Can you work these out from the drawing? Everything is in mm from the part's minimum corner. A direction names the side the tool comes from. Round coordinates to 2 decimals unless told otherwise and drop trailing zeros. Order: outer loops, then holes, each group sorted by start corner. A loop starts at its lowest first (then second) coordinate and runs counter-clockwise, first axis right, second up. Notation, with made-up numbers: (8.25, 71.5) - (43.25, 71.5) arc R23 ccw to (43.25, 98.5) - close; hole circle Ø8 at (50.5, 21.5). An arc over 180 degrees is marked (long way). Answer as a JSON object with one key per item and string values.
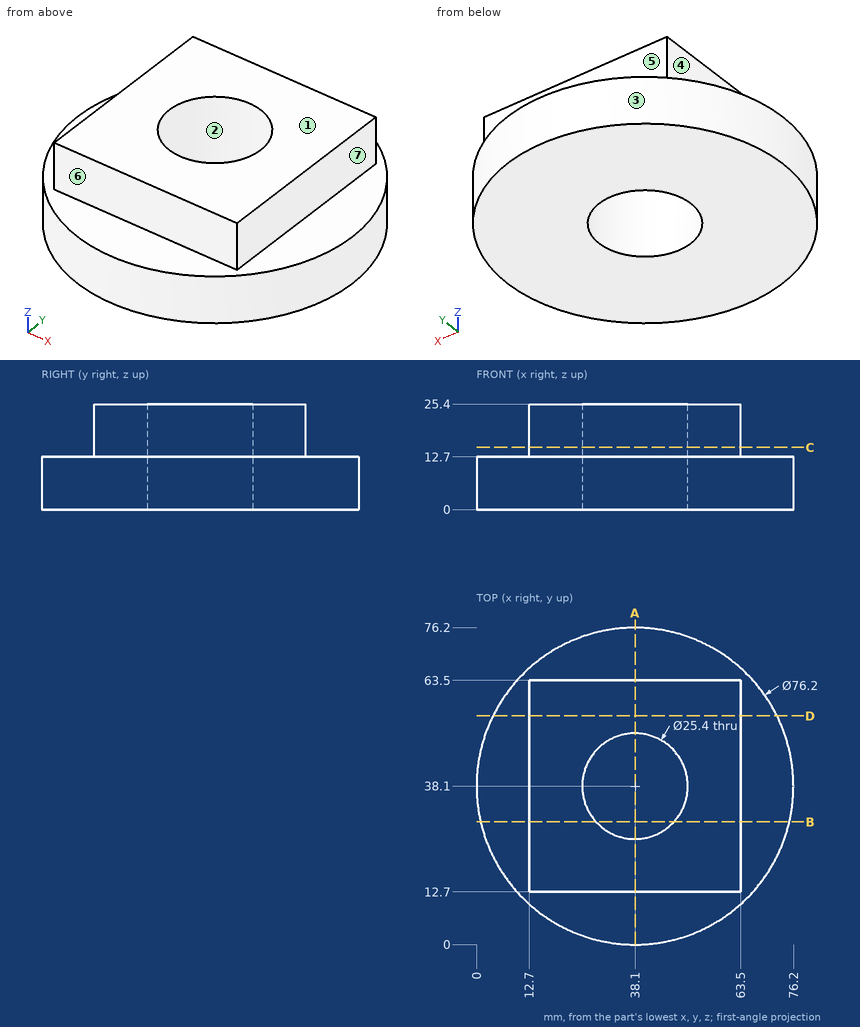
1. Imagine slicing it at A-A (x = 38.1). List the corners of the cut face in (y, z) for me.
Responses:
{"outline": "(0, 0) - (25.4, 0) - (25.4, 25.4) - (12.7, 25.4) - (12.7, 12.7) - (0, 12.7) - close; (50.8, 0) - (76.2, 0) - (76.2, 12.7) - (63.5, 12.7) - (63.5, 25.4) - (50.8, 25.4) - close"}
2. Imagine slicing it at D-D (y = 55). List the corners of the cut face in (x, z) for me.
Responses:
{"outline": "(3.95, 0) - (72.25, 0) - (72.25, 12.7) - (63.5, 12.7) - (63.5, 25.4) - (12.7, 25.4) - (12.7, 12.7) - (3.95, 12.7) - close"}
3. For the marked faces 4, 5, 6 and 7, which set-ups out of +Z, -Z, +X, -X, +Y, -Y let a thin tool reach every point of the face, with its end or its side?
Responses:
{"face 4": "+Z, -X, +Y, -Y", "face 5": "+Z, +X, -X, +Y", "face 6": "+Z, +X, -X, -Y", "face 7": "+Z, +X, +Y, -Y"}
4. Imagine slicing it at C-C (z = 15). List the corners of the cut face in (x, y) for me, plus the area to 3 significant figures.
Responses:
{"outline": "(12.7, 12.7) - (63.5, 12.7) - (63.5, 63.5) - (12.7, 63.5) - close; hole circle Ø25.4 at (38.1, 38.1)", "area": "2,070 mm2"}
5. Imagine slicing it at B-B (y = 29.5). List the corners of the cut face in (x, z) for me.
Responses:
{"outline": "(0.98, 0) - (28.75, 0) - (28.75, 25.4) - (12.7, 25.4) - (12.7, 12.7) - (0.98, 12.7) - close; (47.45, 0) - (75.22, 0) - (75.22, 12.7) - (63.5, 12.7) - (63.5, 25.4) - (47.45, 25.4) - close"}
6. For P1, Ø12, axis at x = 11.5, z = 9.5, coming from the +Y side; P2, Ø1, axis at x = 22, z = 4.5, coming from the +Y side; P3, Ø4, axis at x = 37.5, z = 22, coming from the +Y side; P4, Ø8, axis at x = 9, y = 50.5, coming from the +Z side, each with a flat end and sliding along its axis, tell me the tip position at first contact or that it passes through.
Responses:
{"P1": "y = 70.15", "P2": "y = 72.86", "P3": "y = 63.5", "P4": "z = 25.4"}
7. Thinking about a two-plate mould opening in Y: for the marked faces 1, 2 and 3, which applies, pulls with the +Y half, pulls with the -Y half, needs draft (parallel to the pull), parting line crosses it, or undercut?
Responses:
{"face 1": "needs draft", "face 2": "undercut", "face 3": "parting line crosses it"}
8. If I drill on L1, parallel to X at y = 37.5, z = 19; L2, parallel to Y at x = 38.1, z = 20.25; L3, parallel to Y at x = 47.5, z = 5.5, over which ranges is the centre line in solid material (lowest first)? Write a range as [from, to].
Responses:
{"L1": "[12.7, 25.41], [50.79, 63.5]", "L2": "[12.7, 25.4], [50.8, 63.5]", "L3": "[1.18, 29.56], [46.64, 75.02]"}
